Build history of the part. All positions in model axes, mm. Give positions to 0.01 mm unless a question says otherwise; leave off trailing zeros. Loops run counter-clockwise (first coordinate to the right, second up) from the corner with the lowest first, then second, coordinate; pieces in that order, holes last.
1) Flat gauge pins, fed straight in: P1, Ø0.6, axis at x = 20, y = 1, coming from the +Z side; P2, Ø1.6, axis at x = 86, y = -2.5, coming from the -Z side; P3, Ø0.9, axis at y = -3, z = 9, coming from the -X side. Where does each tip first touch, or does it go through?
2) Band-saw the part on A-A on x = 136. List the corners of the cut face in (y, z).
3) Wall check: line 1 (X direction, y = 0.7, z = 0) (3 decimals); line 2 (X direction, y = 0.5, z = 3); line 3 (Z direction, x = 32.5, y = -5). Give the ranges that are in metal, low to high.
4) Band-saw the part on B-B on x = 0. List the corners of the cut face in (y, z) (3 decimals).
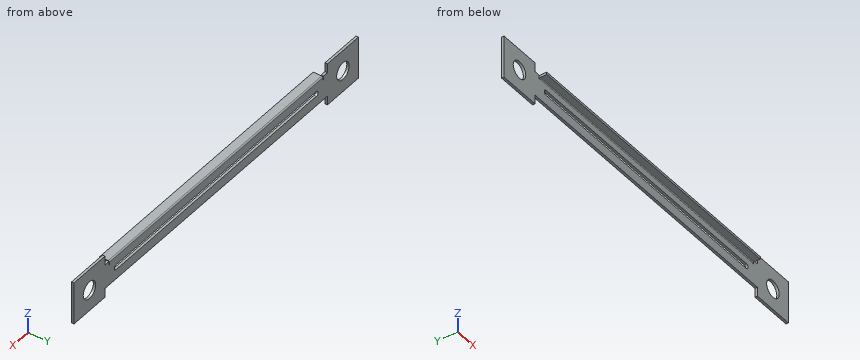
```python
from build123d import *

# Parameters (mm, degrees)
SKETCH1_R           = 7.075
BOSS_EXTRUDE1_DEPTH = 2
SKETCH2_W           = 241
SKETCH2_H           = 2
BOSS_EXTRUDE2_DEPTH = 6
SKETCH3_W           = 0.5
SKETCH3_H           = 2
CUT_EXTRUDE1_DEPTH  = 3
FILLET1_R           = 1
FILLET2_R           = 0.7
CUT_EXTRUDE2_DEPTH  = 305.063315775


with BuildPart() as part:
    # Sketch1 → Boss-Extrude1 (new body)
    with BuildSketch(Plane(origin=(0, 0, 0), x_dir=(1, 0, 0), z_dir=(0, 1, 0))):
        Polygon((-17.5, 17.5), (17.5, 17.5), (17.5, 10), (268.5, 10), (268.5, 17.5), (303.5, 17.5), (303.5, -17.5), (268.5, -17.5), (268.5, -10), (17.5, -10), (17.5, -17.5), (-17.5, -17.5), align=None)
        with Locations(Location((0, 0, 0), (0, 0, 270))):
            Circle(SKETCH1_R, mode=Mode.SUBTRACT)
        with Locations(Location((286, 0, 0), (0, 0, 270))):
            Circle(SKETCH1_R, mode=Mode.SUBTRACT)
    extrude(amount=BOSS_EXTRUDE1_DEPTH)

    # Sketch2 → Boss-Extrude2 (add)
    with BuildSketch(Plane.XZ):
        with Locations((143, 9)):
            Rectangle(SKETCH2_W, SKETCH2_H)
    extrude(amount=BOSS_EXTRUDE2_DEPTH)

    # Sketch3 → Cut-Extrude1 (cut)
    with BuildSketch(Plane.XY.offset(10)):
        with Locations((22.25, 1)):
            Rectangle(SKETCH3_W, SKETCH3_H)
        with Locations((263.75, 1)):
            Rectangle(SKETCH3_W, SKETCH3_H)
    extrude(amount=-CUT_EXTRUDE1_DEPTH, mode=Mode.SUBTRACT)

    # Fillet1
    fillet1_edges = [part.edges().sort_by_distance(p)[0] for p in [
        (143, 2, 10),
    ]]
    fillet(fillet1_edges, radius=FILLET1_R)

    # Fillet2
    fillet2_edges = [part.edges().sort_by_distance(p)[0] for p in [
        (143, 0, 8),
    ]]
    fillet(fillet2_edges, radius=FILLET2_R)

    # Sketch4 → Cut-Extrude2 (cut, through all)
    with BuildSketch(Plane.XZ):
        with BuildLine():
            Line((30, 2.05), (256, 2.05))
            ThreePointArc((256, 2.05), (258.05, 0), (256, -2.05))
            Line((256, -2.05), (30, -2.05))
            ThreePointArc((30, -2.05), (27.95, 0), (30, 2.05))
        make_face()
    extrude(amount=-CUT_EXTRUDE2_DEPTH, mode=Mode.SUBTRACT)


solid = part.part
```
Findings below:
1. P1: stops at z = 10
1. P2: stops at z = 8
1. P3: stops at x = 22.5
2. outline: (-6, 8) - (-0.7, 8) arc R0.7 cw to (0, 7.3) - (0, 2.05) - (2, 2.05) - (2, 9) arc R1 ccw to (1, 10) - (-6, 10) - close; (0, -10) - (2, -10) - (2, -2.05) - (0, -2.05) - close
3. line 1: x = -17.5 to -7.075, 7.075 to 27.95, 258.05 to 278.925, 293.075 to 303.5
3. line 2: x = -17.5 to -6.41, 6.41 to 279.59, 292.41 to 303.5
3. line 3: z = 8 to 10
4. outline: (0, -17.5) - (2, -17.5) - (2, -7.075) - (0, -7.075) - close; (0, 7.075) - (2, 7.075) - (2, 17.5) - (0, 17.5) - close
